Geometry check sheet. Reference: the model listing, model coordinates, mm. A direction names the side the tool comes from. Coordinates: 2 decimals unless noted, no trailing zeros. Loops run counter-clockwise (first coordinate to the right, second up) from the corner with the lowest first, then second, coordinate; pieces in that order, holes last.
from build123d import *

# Parameters (mm, degrees)
BOSS_EXTRUDE1_DEPTH   = 5
BOSS_EXTRUDE1_2_DEPTH = 5
SKETCH1_3_W           = 3.760900756
SKETCH1_3_H           = 5
SKETCH1_3_W_2         = 25.78972556
BOSS_EXTRUDE2_DEPTH   = 7
CUT_EXTRUDE1_REACH    = 12.869
SKETCH2_R             = 1.1
SKETCH3_R             = 2
CUT_EXTRUDE2_DEPTH    = 4


with BuildPart() as part:
    # Sketch1 → Boss-Extrude1 (new body, symmetric)
    with BuildSketch(Plane.XY):
        with BuildLine():
            Line((12.89486278, 5.341227048), (12.89486278, 2.5))
            Line((12.89486278, 2.5), (16.655763536, 2.5))
            Line((16.655763536, 2.5), (16.655763536, -2.5))
            Line((16.655763536, -2.5), (12.89486278, -2.5))
            Line((12.89486278, -2.5), (12.89486278, -5.341227048))
            Line((12.89486278, -5.341227048), (20.204359293, -8.368919638))
            ThreePointArc((20.204359293, -8.368919638), (21.869040911, 0), (20.204359293, 8.368919638))
            Line((20.204359293, 8.368919638), (12.89486278, 5.341227048))
        make_face()
    extrude(amount=BOSS_EXTRUDE1_DEPTH, both=True)



with BuildPart() as body_2:
    # Sketch1 → Boss-Extrude1 2 (new body, symmetric)
    with BuildSketch(Plane.XY):
        with BuildLine():
            Line((-12.89486278, 5.341227048), (-20.204359293, 8.368919638))
            ThreePointArc((-20.204359293, 8.368919638), (-21.869040911, 0), (-20.204359293, -8.368919638))
            Line((-20.204359293, -8.368919638), (-12.89486278, -5.341227048))
            Line((-12.89486278, -5.341227048), (-12.89486278, -2.5))
            Line((-12.89486278, -2.5), (-16.655763536, -2.5))
            Line((-16.655763536, -2.5), (-16.655763536, 2.5))
            Line((-16.655763536, 2.5), (-12.89486278, 2.5))
            Line((-12.89486278, 2.5), (-12.89486278, 5.341227048))
        make_face()
    extrude(amount=BOSS_EXTRUDE1_2_DEPTH, both=True)


with BuildPart() as part_1:
    add(part.part)

    add(body_2.part)  # Boss-Extrude2 merges body 2
    # Sketch1_3 → Boss-Extrude2 (add, symmetric)
    with BuildSketch(Plane.XY):
        with Locations((14.775313158, 0)):
            Rectangle(SKETCH1_3_W, SKETCH1_3_H)
        Rectangle(SKETCH1_3_W_2, SKETCH1_3_H)
        with Locations((-14.775313158, 0)):
            Rectangle(SKETCH1_3_W, SKETCH1_3_H)
    extrude(amount=BOSS_EXTRUDE2_DEPTH, both=True)

    # Sketch2 → Cut-Extrude1 (cut, up to next)
    with BuildSketch(Plane(origin=(0, 2.5, 0), x_dir=(1, 0, 0), z_dir=(0, 1, 0)), mode=Mode.PRIVATE) as cut_extrude1_sk1:
        Circle(SKETCH2_R)
    cut_extrude1_tool1 = extrude(cut_extrude1_sk1.sketch, amount=-CUT_EXTRUDE1_REACH, mode=Mode.PRIVATE) & part_1.part
    add(cut_extrude1_tool1.solids().sort_by_distance((0, 2.5, 0))[0], mode=Mode.SUBTRACT)

    # Sketch3 → Cut-Extrude2 (cut)
    with BuildSketch(Plane(origin=(21.869040911, 0, 0), x_dir=(0, 0, -1), z_dir=(1, 0, 0))):
        Circle(SKETCH3_R)
    cut_extrude2 = extrude(amount=-CUT_EXTRUDE2_DEPTH, mode=Mode.SUBTRACT)

    # Mirror1: Cut-Extrude2 across plane
    add(cut_extrude2.mirror(Plane(origin=(0, 0, 0), x_dir=(0, 0, 1), z_dir=(1, 0, 0))), mode=Mode.SUBTRACT)


solid = part_1.part
(1) Access from +Z, -Z, +X, -X, +Y, -Y to the whole of each face (thin tool, end or side, straight path). Record for faces 1 (the cylindrical face through (-20, -2, 0)), 2 (the flat face through (-16.656, 0, 6)), 3 (the flat face through (16.498, -6.834, 0.07)), 4 (the flat face through (-16.656, 0, -6)), 5 (the flat face through (16.656, 0, 6)).
Findings:
face 1: -X
face 2: +Z, -X, +Y, -Y
face 3: +Z, -Z, -Y
face 4: -Z, -X, +Y, -Y
face 5: +Z, +X, +Y, -Y
(2) Scan lines: L1, parallel to Z at x = 0, y = 0.2; L2, parallel to Z at x = -20.5, y = 0; L3, parallel to X at y = -1.1, z = 0. Record each from-to range of solid material in increasing order.
Findings:
L1: z = -7 to -1.1, 1.1 to 7
L2: z = -5 to -2, 2 to 5
L3: x = -17.87 to -1.1, 1.1 to 17.87
(3) Gauge pin test, flat ends, axial feed: pin 1 Ø1 at (y, z) = (3.5, -3.5) entering from -X; pin 2 Ø4 at (y, z) = (-2.5, -2) entering from +X; pin 3 Ø2 at (y, z) = (-0.5, 6.5) entering from +X. Record the tip position at first contact, or that the pin passes through.
Findings:
pin 1: stops at x = -21.66
pin 2: stops at x = 21.86
pin 3: stops at x = 16.66
(4) Sectioned sample at D-D on z = 0. Record the cut outline in (x, y).
Findings:
outline: (-21.78, -2) arc R21.87 ccw to (-20.2, -8.37) - (-12.89, -5.34) - (-12.89, -2.5) - (-1.1, -2.5) - (-1.1, 2.5) - (-12.89, 2.5) - (-12.89, 5.34) - (-20.2, 8.37) arc R21.87 ccw to (-21.78, 2) - (-17.87, 2) - (-17.87, -2) - close; (1.1, -2.5) - (12.89, -2.5) - (12.89, -5.34) - (20.2, -8.37) arc R21.87 ccw to (21.78, -2) - (17.87, -2) - (17.87, 2) - (21.78, 2) arc R21.87 ccw to (20.2, 8.37) - (12.89, 5.34) - (12.89, 2.5) - (1.1, 2.5) - close
(5) Sectioned sample at B-B on y = 0. Record the cut outline in (x, z), and give its area (3 significant figures).
Findings:
outline: (-21.87, -5) - (-16.66, -5) - (-16.66, -7) - (16.66, -7) - (16.66, -5) - (21.87, -5) - (21.87, -2) - (17.87, -2) - (17.87, 2) - (21.87, 2) - (21.87, 5) - (16.66, 5) - (16.66, 7) - (-16.66, 7) - (-16.66, 5) - (-21.87, 5) - (-21.87, 2) - (-17.87, 2) - (-17.87, -2) - (-21.87, -2) - close; hole circle Ø2.2 at (0, 0)
area: 535 mm2
(6) Draft check along X on faces 6 (the flat face through (-18, 0, 5)), 7 (the flat face through (-17.869, 0, 0)), 8 (the flat face through (0, -2.5, 2)). Enter one of: +X half, -X half, draft (parallel to the pull), parting line (faces both ways), or undercut.
Findings:
face 6: draft
face 7: -X half
face 8: undercut
(7) Sectioned sample at A-A on x = 0. Record the cut outline in (y, z).
Findings:
outline: (-2.5, -7) - (2.5, -7) - (2.5, -1.1) - (-2.5, -1.1) - close; (-2.5, 1.1) - (2.5, 1.1) - (2.5, 7) - (-2.5, 7) - close
(8) Sectioned sample at C-C on y = -4. Record the cut outline in (x, z), and give its area (3 significant figures).
Findings:
outline: (-21.5, -5) - (-12.89, -5) - (-12.89, 5) - (-21.5, 5) - close; (12.89, -5) - (21.5, -5) - (21.5, 5) - (12.89, 5) - close
area: 172 mm2
